The listing builds one solid part. Answer for the finished solid, in the listing's coordinates (mm). A direction names the side the tool comes from. Coordinates: 2 decimals unless noted, no trailing zeros. Write each loop counter-clockwise with the first axis right and the second up, starting at its lowest first coordinate (ties: lowest second). Pieces come first, ordered by that corner, then holes.
from build123d import *

# Parameters (mm, degrees)
EXTRUDE_1_DEPTH     = 20
SKETCH_2_R          = 2.75
SKETCH_2_R_2        = 4
CUT_EXTRUDE_1_DEPTH = 75.303431953
SKETCH_3_R          = 12.5
CUT_EXTRUDE_2_DEPTH = 3
SKETCH_4_R          = 2.75
CUT_EXTRUDE_3_DEPTH = 72.107313267
SKETCH_5_R          = 6
CUT_EXTRUDE_4_DEPTH = 6


with BuildPart() as part:
    # Эскиз1 → Бобышка-Вытянуть1 (new body)
    with BuildSketch(Plane.XY):
        Polygon((47, 32.5), (60, 32.5), (60, 0), (0, 0), (0, 32.5), (13, 32.5), (13, 39), (47, 39), align=None)
    extrude(amount=EXTRUDE_1_DEPTH)

    # Эскиз2 → Вырез-Вытянуть1 (cut, through all)
    with BuildSketch(Plane.XY.offset(20)):
        with Locations((7, 22)):
            Circle(SKETCH_2_R)
        with Locations((7, 7)):
            Circle(SKETCH_2_R)
        with Locations((53, 22)):
            Circle(SKETCH_2_R)
        with Locations((53, 7)):
            Circle(SKETCH_2_R)
        with Locations((30, 22)):
            Circle(SKETCH_2_R_2)
    extrude(amount=-CUT_EXTRUDE_1_DEPTH, mode=Mode.SUBTRACT)

    # Эскиз3 → Вырез-Вытянуть2 (cut)
    with BuildSketch(Plane.XY.offset(20)):
        with Locations((30, 22)):
            Circle(SKETCH_3_R)
    extrude(amount=-CUT_EXTRUDE_2_DEPTH, mode=Mode.SUBTRACT)

    # Эскиз4 → Вырез-Вытянуть3 (cut, through all)
    with BuildSketch(Plane(origin=(0, 32.5, 0), x_dir=(1, 0, 0), z_dir=(0, 1, 0))):
        with Locations(Location((7, -10, 0), (0, 0, 180))):
            Circle(SKETCH_4_R)
        with Locations(Location((53, -10, 0), (0, 0, 180))):
            Circle(SKETCH_4_R)
    extrude(amount=-CUT_EXTRUDE_3_DEPTH, mode=Mode.SUBTRACT)

    # Эскиз5 → Вырез-Вытянуть4 (cut)
    with BuildSketch(Plane(origin=(0, 32.5, 0), x_dir=(1, 0, 0), z_dir=(0, 1, 0))):
        with Locations(Location((7, -10, 0), (0, 0, 180))):
            Circle(SKETCH_5_R)
        with Locations(Location((53, -10, 0), (0, 0, 180))):
            Circle(SKETCH_5_R)
    extrude(amount=-CUT_EXTRUDE_4_DEPTH, mode=Mode.SUBTRACT)


solid = part.part
Q1. Given pin 1 (3 mm diameter, centred on x = 28, y = 6.5, fed in from -Z); pin 2 (3.5 mm diameter, centred on x = 51, z = 7.5, fed in from +Y); pin 3 (1.5 mm diameter, centred on x = 27.5, y = 13, fed in from +Z); pin 4 (9.5 mm diameter, centred on x = 4, z = 9.5, fed in from +Y), each flat-ended and moving along its own axis, determine where each tip first touches the part or whether it passes through.
Answers below:
pin 1: stops at z = 0
pin 2: stops at y = 26.5
pin 3: stops at z = 17
pin 4: stops at y = 32.5
Q2. The part is cut by section D-D, the plane y = 8. Write down the section's boundary in (x, z), then the cut area to 3 significant figures.
Answers below:
outline: (0, 0) - (4.44, 0) - (4.44, 9) arc R2.75 cw to (4.44, 11) - (4.44, 20) - (0, 20) - close; (9.56, 0) - (50.44, 0) - (50.44, 9) arc R2.75 cw to (50.44, 11) - (50.44, 20) - (9.56, 20) - (9.56, 11) arc R2.75 cw to (9.56, 9) - close; (55.56, 0) - (60, 0) - (60, 20) - (55.56, 20) - (55.56, 11) arc R2.75 cw to (55.56, 9) - close
area: 994 mm2
Q3. Which of the six approach directions +Z, -Z, +X, -X, +Y, -Y give full straight-line access (tool end or side, diameter ignored) to faces 4 (the face through (50, 26.5, 9)), 5 (the face through (59.2, 32.5, 9.9)), 6 (the face through (27, 25, 17)), 7 (the face through (0.6, 32.5, 9.9)), 8 (the face through (4.818, 20.327, 16.181))?
Answers below:
face 4: +Y
face 5: +Z, -Z, +X, +Y
face 6: +Z
face 7: +Z, -Z, -X, +Y
face 8: +Z, -Z
Q4. Find the intervals of material crossed by probe 1 along Y at (x, z) = (7, 14.5); probe 2 along Y at (x, z) = (30, 2.5); probe 3 along X at (y, z) = (19.5, 14), in increasing order.
Answers below:
probe 1: y = 0 to 4.25, 9.75 to 19.25, 24.75 to 26.5
probe 2: y = 0 to 18, 26 to 39
probe 3: x = 0 to 5.85, 8.15 to 26.88, 33.12 to 51.85, 54.15 to 60
Q5. The part is cut by section A-A, the plane x = 53. Write down the section's boundary in (y, z), then the cut area to 3 significant figures.
Answers below:
outline: (0, 0) - (4.25, 0) - (4.25, 7.25) - (0, 7.25) - close; (0, 12.75) - (4.25, 12.75) - (4.25, 20) - (0, 20) - close; (9.75, 0) - (19.25, 0) - (19.25, 7.25) - (9.75, 7.25) - close; (9.75, 12.75) - (19.25, 12.75) - (19.25, 20) - (9.75, 20) - close; (24.75, 0) - (32.5, 0) - (32.5, 4) - (26.5, 4) - (26.5, 7.25) - (24.75, 7.25) - close; (24.75, 12.75) - (26.5, 12.75) - (26.5, 16) - (32.5, 16) - (32.5, 20) - (24.75, 20) - close
area: 273 mm2
Q6. The part is cut by section C-C, the plane y = 14. Write down the section's boundary in (x, z), then the cut area to 3 significant figures.
Answers below:
outline: (0, 0) - (60, 0) - (60, 20) - (39.6, 20) - (39.6, 17) - (20.4, 17) - (20.4, 20) - (0, 20) - close; hole circle Ø5.5 at (7, 10); hole circle Ø5.5 at (53, 10)
area: 1,090 mm2
Q7. The part is cut by section B-B, the plane z = 17.75. Write down the section's boundary in (x, y), then the cut area to 3 significant figures.
Answers below:
outline: (0, 0) - (60, 0) - (60, 32.5) - (47, 32.5) - (47, 39) - (13, 39) - (13, 32.5) - (0, 32.5) - close; hole circle Ø5.5 at (7, 7); hole circle Ø5.5 at (7, 22); hole circle Ø25 at (30, 22); hole circle Ø5.5 at (53, 7); hole circle Ø5.5 at (53, 22)
area: 1,590 mm2
Q8. Determine the mould class of faces 1 (the face through (55.027, 14.605, 11.859)), 2 (the face through (30, 39, 10)), 3 (the face through (20.08, 14.394, 18.521)) for opening direction Y: released by +Y, released by -Y, zero draft, split by the parting line, or undercut.
Answers below:
face 1: zero draft
face 2: released by +Y
face 3: undercut
